The model under review builds one solid part; all positions refer to its coordinate system, in mm. Face numbers are marked on the shaded views. A direction names the side the tool comes from. Round coordinates to 2 decimals unless told otherwise and drop trailing zeros. Write each loop counter-clockwise with the first axis right and the second up, starting at its lowest first coordinate (ties: lowest second). Pieces come first, ordered by that corner, then holes. Notation, with made-up numbers: (-0.75, 87) - (38.25, 87) arc R28 ccw to (38.25, 105) - close; hole circle Ø3 at (8.25, -9.75). An arc over 180 degrees is marked (long way). Return JSON: item names as keys, results as strings.
from build123d import *

# Parameters (mm, degrees)
F1_DEPTH = 127
F3_DEPTH = 127


with BuildPart() as f1:
    # F0 (on Front) → F1 (new body)
    with BuildSketch(Plane.XZ):
        Polygon((-89.792244, 54.44082), (-89.792244, -47.15918), (62.607756, -47.15918), (62.607756, 54.44082), (37.207756, 54.44082), (37.207756, 3.64082), (-64.392244, 3.64082), (-64.392244, 54.44082), align=None)
    extrude(amount=F1_DEPTH)

    # F2 (on Top) → F3 (join)
    with BuildSketch(Plane.XY):
        Polygon((11.475189, 50.8), (-140.924811, 50.8), (-140.924811, -76.2), (-115.524811, -76.2), (-115.524811, 0), (-13.924811, 0), (-13.924811, -76.2), (11.475189, -76.2), align=None)
    extrude(amount=F3_DEPTH)


solid = f1.part
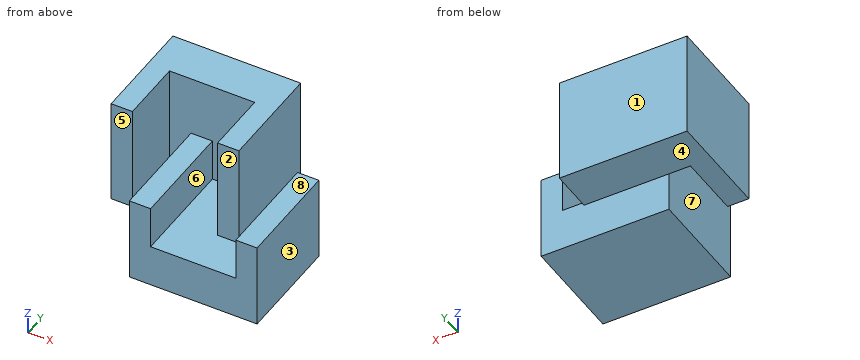
(1) Clearance check with flat-ended pins moving along their axes: pin 1 Ø2 at (y, z) = (-105.5, 43) entering from -X; pin 2 Ø5 at (y, z) = (-4, 109.5) entering from +X; pin 3 Ø1.5 at (x, z) = (33, -28) entering from +Y. State where each tip first meets the part, or that it passes through.
Filled in:
{"pin 1": "stops at x = -89.79", "pin 2": "stops at x = 11.48", "pin 3": "stops at y = 0"}
(2) For the marked faces 4, 5, 6, 7 and 8, list the 3-axis set-ups (+Z, -Z, +X, -X, +Y, -Y) from which the entire face can be reached by the end or side of a thin tool; tool diameter is ignored.
Filled in:
{"face 4": "-Z, -X, +Y", "face 5": "+Z, -Z, -X, -Y", "face 6": "+Z, -Y", "face 7": "+Z, -Z, -Y", "face 8": "+Z, +X, +Y, -Y"}
(3) Add section D-D (z = 113). Write out the cut boundary in (x, y), plus the area to 3 significant figures.
Filled in:
{"outline": "(-140.92, -76.2) - (-115.52, -76.2) - (-115.52, 0) - (-13.92, 0) - (-13.92, -76.2) - (11.48, -76.2) - (11.48, 50.8) - (-140.92, 50.8) - close", "area": "11,600 mm2"}
(4) Mouldability with a two-part tool opening along X and no side actions: class the marked faces 1, 2 and 3 as released by +X, released by -X, zero draft, split by the parting line, or undercut.
Filled in:
{"face 1": "zero draft", "face 2": "undercut", "face 3": "released by +X"}
(5) Add section B-B (y = -54.5). Write out the cut boundary in (x, z).
Filled in:
{"outline": "(-140.92, 0) - (-115.52, 0) - (-115.52, 127) - (-140.92, 127) - close; (-89.79, -47.16) - (62.61, -47.16) - (62.61, 54.44) - (37.21, 54.44) - (37.21, 3.64) - (11.48, 3.64) - (11.48, 127) - (-13.92, 127) - (-13.92, 3.64) - (-64.39, 3.64) - (-64.39, 54.44) - (-89.79, 54.44) - close"}
(6) Add section C-C (x = -32). Write out the cut boundary in (y, z), plus the area to 3 significant figures.
Filled in:
{"outline": "(-127, -47.16) - (0, -47.16) - (0, 0) - (50.8, 0) - (50.8, 127) - (0, 127) - (0, 3.64) - (-127, 3.64) - close", "area": "12,900 mm2"}
(7) Add section A-A (z = 30). Write out the cut boundary in (x, y), plus the area to 3 significant figures.
Filled in:
{"outline": "(-140.92, -76.2) - (-115.52, -76.2) - (-115.52, 0) - (-89.79, 0) - (-89.79, -127) - (-64.39, -127) - (-64.39, 0) - (-13.92, 0) - (-13.92, -76.2) - (11.48, -76.2) - (11.48, 50.8) - (-140.92, 50.8) - close; (37.21, -127) - (62.61, -127) - (62.61, 0) - (37.21, 0) - close", "area": "18,100 mm2"}
(8) Wall thickness on line 1 (X direction, y = -49.5, z = 40); line 2 (X direction, y = -97, z = 30.5); line 3 (Y direction, x = 9, z = 97): over which ranges is each line inside the solid? List them lowest first.
Filled in:
{"line 1": "x = -140.92 to -115.52, -89.79 to -64.39, -13.92 to 11.48, 37.21 to 62.61", "line 2": "x = -89.79 to -64.39, 37.21 to 62.61", "line 3": "y = -76.2 to 50.8"}
